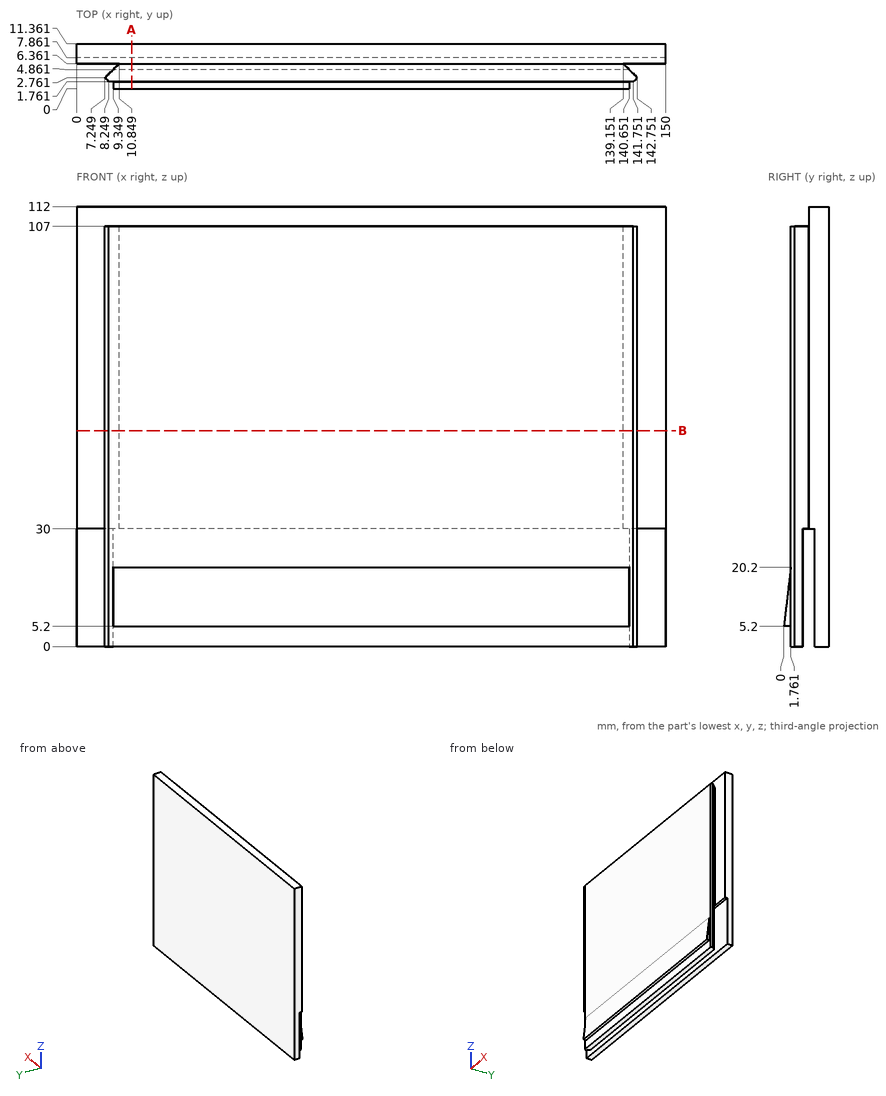
Print and shaded views of the part. All mm, measured from the part's lowest x, y and z. Coordinates: 2 decimals unless noted, no trailing zeros. Loops run counter-clockwise (first coordinate to the right, second up) from the corner with the lowest first, then second, coordinate; pieces in that order, holes last. Notation, with made-up numbers: M 9,-14 L 64,-14 A12 ccw 64,3 Z; hole C 9.5,-30 d11. An arc over 180 degrees is marked long. Use a Markdown table: item, result. Add a question column.
Q1. Cut at B-B (z = 55). Write the cut outline in (x, y), and give its area (3 significant figures).
Q2. Cut at A-A (x = 14). Write the cut outline in (y, z).
Q3. Probe L1, parallel to Y at x = 51.5, z = 5; L2, parallel to Y at x = 87.5, z = 104.5; L3, parallel to Z at x = 60.5, y = 5. List the from-to ranges inside material, lowest first.
Q4. Pin check, flat tips, straight feed: P1, Ø6, axis at x = 120, z = 32.5, coming from the -Y side; P2, Ø2.5, axis at x = 94, y = 3.5, coming from the +Z side; P3, Ø1.9, axis at y = 1, z = 13.5, coming from the -X side. Stop position of each tip, or through.
Worked out:
| question | item | result |
|---|---|---|
| 1 | outline | M 0,6.36 L 10.85,6.36 L 7.25,2.76 L 8.25,1.76 L 141.75,1.76 L 142.75,2.76 L 139.15,6.36 L 150,6.36 L 150,11.36 L 0,11.36 Z |
| 1 | area | 1,360 mm2 |
| 2 | outline | M 0,5.2 L 1.76,5.2 L 1.76,0 L 4.86,0 L 4.86,30 L 7.86,30 L 7.86,0 L 11.36,0 L 11.36,112 L 6.36,112 L 6.36,107 L 1.76,107 L 1.76,20.2 Z |
| 3 | L1 | y = 1.76 to 4.86, 7.86 to 11.36 |
| 3 | L2 | y = 1.76 to 11.36 |
| 3 | L3 | z = 30 to 107 |
| 4 | P1 | stops at y = 1.76 |
| 4 | P2 | stops at z = 107 |
| 4 | P3 | stops at x = 8.06 |
